from build123d import *

# Parameters (mm, degrees)
F0_R     = 6.35
F1_DEPTH = 25.4
F2_W     = 39.37
F2_H     = 25.4
F3_DEPTH = 25.4
F5_DEPTH = 25.4
F6_W     = 15.24
F6_H     = 2.54
F7_DEPTH = 57.15
F8_W     = 7.62
F8_H     = 1.016
F9_DEPTH = 35.56


with BuildPart() as f1:
    # F0 (on Front) → F1 (new body)
    with BuildSketch(Plane.XZ):
        Circle(F0_R)
    extrude(amount=F1_DEPTH)

    # F2 (on face) → F3 (join)
    with BuildSketch(Plane.XZ.offset(25.4)):
        Rectangle(F2_W, F2_H)
    extrude(amount=F3_DEPTH)

    # F4 (on face) → F5 (cut)
    with BuildSketch(Plane.XY.offset(12.7)):
        with BuildLine():
            Line((-4.445, -33.1953875721), (-4.445, -50.8))
            Line((-4.445, -50.8), (4.445, -50.8))
            Line((4.445, -50.8), (4.445, -33.1953875721))
            ThreePointArc((4.445, -33.1953875721), (0, -37.6403875721), (-4.445, -33.1953875721))
        make_face()
        with BuildLine():
            ThreePointArc((4.445, -33.1953875721), (0, -28.7503875721), (-4.445, -33.1953875721))
            Line((-4.445, -33.1953875721), (4.445, -33.1953875721))
        make_face()
        with BuildLine():
            Line((4.445, -33.1953875721), (-4.445, -33.1953875721))
            ThreePointArc((-4.445, -33.1953875721), (0, -37.6403875721), (4.445, -33.1953875721))
        make_face()
    extrude(amount=-F5_DEPTH, mode=Mode.SUBTRACT)

    # F6 (on face) → F7 (join)
    with BuildSketch(Plane.XZ.offset(50.8)):
        with Locations((-12.065, -11.43)):
            Rectangle(F6_W, F6_H)
        with Locations((12.065, -11.43)):
            Rectangle(F6_W, F6_H)
    extrude(amount=F7_DEPTH)

    # F8 (on face) → F9 (cut)
    with BuildSketch(Plane.YZ.offset(19.685)):
        with Locations((-103.124, -11.43)):
            Rectangle(F8_W, F8_H)
    extrude(amount=-F9_DEPTH, mode=Mode.SUBTRACT)


solid = f1.part
Verification items for the finished model (mm, model axes). A direction names the side the tool comes from. Coordinates: 2 decimals unless noted, no trailing zeros. Write each loop counter-clockwise with the first axis right and the second up, starting at its lowest first coordinate (ties: lowest second). Pieces come first, ordered by that corner, then holes. Notation, with made-up numbers: M 19,-26.5 L 68,-26.5 A17 ccw 68,-17.5 Z; hole C -34.75,66 d6. An arc over 180 degrees is marked long. Use CSV: the item, a comma, the result in double quotes.
Q1. Section check A-A, the plane y = -90. Enter the section's corners in (x, z) (3 decimals), and give its area (3 significant figures).
Computed values:
outline,"M -19.685,-12.7 L -4.445,-12.7 L -4.445,-10.16 L -19.685,-10.16 Z; M 4.445,-12.7 L 19.685,-12.7 L 19.685,-10.16 L 4.445,-10.16 Z"
area,"77.4 mm²"
Q2. Set-up check for faces 5 (the flat face through (4.445, -49, -4)), 6 (the flat face through (-5, -38, 12.7)), 7 (the cylindrical face through (-1.38, -12.52, -6.2)), 8 (the flat face through (-10, -103, -10.922)), 9 (the flat face through (-12, -79, -10.16)): record each of +Z, -Z, +X, -X, +Y, -Y from which the full face is reachable in a straight line by a thin tool's end or side.
Computed values:
face 5,"+Z, -Z, -Y"
face 6,"+Z, +X, -X, +Y, -Y"
face 7,"+Y"
face 8,"+X"
face 9,"+Z, +X, -X, -Y"
Q3. Go/stop test with flat-tipped pins: P1, Ø0.8, axis at x = 12, z = -11.5, coming from the +Y side; P2, Ø7.5, axis at x = -16, z = 3, coming from the -Y side; P3, Ø4, axis at x = -11, y = -103.5, coming from the +Z side. Record where each tip stops, or that it passes through.
Computed values:
P1,"y = -25.4"
P2,"y = -50.8"
P3,"z = -10.16"
Q4. Thickness scan on line 1 along Y through (x, z) = (-7, -11.25); line 2 along X through (y, z) = (-39.5, -1.5) (3 decimals); line 3 along Z through (x, y) = (8.5, -99.5). Record the ranges inside material, lowest first. Write a range as [from, to].
Computed values:
line 1,"[-107.95, -106.93], [-99.31, -25.4]"
line 2,"[-19.685, -4.445], [4.445, 19.685]"
line 3,"[-12.7, -11.94], [-10.92, -10.16]"
Q5. Section check C-C, the plane z = 9.25. Enter the section's corners in (x, y) (3 decimals), and give its area (3 significant figures).
Computed values:
outline,"M -19.685,-50.8 L -4.445,-50.8 L -4.445,-33.195 A4.445 cw 4.445,-33.195 L 4.445,-50.8 L 19.685,-50.8 L 19.685,-25.4 L -19.685,-25.4 Z"
area,"812 mm²"
Q6. Mould release check, pull along Y, two halves, no side actions. Record for faces 1 (the flat face through (-12, -50.8, 1)), 2 (the flat face through (12, -103, -10.922)), 3 (the flat face through (0, 0, 0)), 4 (the flat face through (12, -103, -11.938)): pulls with the +Y half, pulls with the -Y half, needs draft (parallel to the pull), parting line crosses it, or undercut.
Computed values:
face 1,"pulls with the -Y half"
face 2,"undercut"
face 3,"pulls with the +Y half"
face 4,"undercut"
Q7. Section check D-D, the plane x = 0. Enter the section's corners in (y, z), and give its area (3 significant figures).
Computed values:
outline,"M -28.75,-12.7 L -25.4,-12.7 L -25.4,-6.35 L 0,-6.35 L 0,6.35 L -25.4,6.35 L -25.4,12.7 L -28.75,12.7 Z"
area,"408 mm²"
Q8. Section check B-B, the plane x = -9.5. Enter the section's corners in (y, z), and give its area (3 significant figures).
Computed values:
outline,"M -107.95,-12.7 L -25.4,-12.7 L -25.4,12.7 L -50.8,12.7 L -50.8,-10.16 L -107.95,-10.16 Z; hole M -106.93,-11.94 L -99.31,-11.94 L -99.31,-10.92 L -106.93,-10.92 Z"
area,"783 mm²"
